Verification items for the finished model (mm, model axes). Face numbers are marked on the shaded views. A direction names the side the tool comes from. Round coordinates to 2 decimals unless told otherwise and drop trailing zeros. Write each loop counter-clockwise with the first axis right and the second up, starting at its lowest first coordinate (ties: lowest second). Pieces come first, ordered by that corner, then holes.
Autodesk Inventor part; units mm, degrees
ref_plane "YZ Plane" through (0, 0, 0) normal (1, 0, 0) x (0, 1, 0)
ref_plane "XZ Plane" through (0, 0, 0) normal (0, 1, 0) x (-1, 0, 0)
ref_plane "XY Plane" through (0, 0, 0) normal (0, 0, 1) x (1, 0, 0)
sketch "Sketch8" plane through (0, 0, 0) normal (0, 0, 1) x (1, 0, 0)
  circle A0 centre (0, 0) radius 15
  dimension "d33" = 30
extrude "Extrusion7" add sketch "Sketch8" against normal blind 8
sketch "Sketch10" plane through (0, 0, -8) normal (0, 0, -1) x (-1, 0, 0)
  line L0 (9, 10.07) -> (-29.1, 10.07)
  arc A0 (10, 9.07) -> (9, 10.07) centre (9, 9.07) ccw
  line L1 (10, 9.07) -> (10, -9.07)
  arc A1 (9, -10.07) -> (10, -9.07) centre (9, -9.07) ccw
  line L2 (-29.1, -10.07) -> (9, -10.07)
  line L3 (-29.1, 10.07) -> (-29.1, -10.07)
  arc A2 (9, -10.47) -> (10.4, -9.07) centre (9, -9.07) ccw
  line L4 (10.4, -9.07) -> (10.4, 9.07)
  arc A3 (10.4, 9.07) -> (9, 10.47) centre (9, 9.07) ccw
  line L5 (9, 10.47) -> (-29.5, 10.47)
  line L6 (-29.5, 10.47) -> (-29.5, -10.47)
  line L7 (-29.5, -10.47) -> (9, -10.47)
  dimension "d59" = 0.4
extrude "Extrusion8" cut sketch "Sketch10" against normal blind 2 contours A0 L1 A1 L2 L3 L0 | L7 L6 L5 A3 L4 A2
sketch "Sketch11" plane through (0, 0, -6) normal (0, 0, -1) x (-1, 0, 0)
  circle A0 centre (0, 0) radius 6.4
  circle A1 centre (0, 0) radius 6.5
  point P0 (0, 0)
  dimension "d58" = 13
extrude "Extrusion9" cut sketch "Sketch11" against normal through all contours A0 | A1
sketch "Sketch13" plane through (0, 0, 0) normal (0, 0, 1) x (1, 0, 0)
  circle A0 centre (0, 0) radius 9.96
  circle A1 centre (0, 0) radius 10.16
  point P0 (0, 0)
  dimension "d44" = 0.2
extrude "Extrusion11" cut sketch "Sketch13" against normal blind 3 contours A0 | A1
sketch "Sketch14" plane through (0, 0, 0) normal (0, 0, 1) x (1, 0, 0)
  circle A0 centre (6.9, 8) radius 0.7835
  circle A1 centre (6.9, -8) radius 0.7835
  circle A2 centre (-8, 8.07) radius 1
  circle A3 centre (-8, -8.07) radius 1
  point P0 (0, 0)
hole "Hole2" at (6.9, 8, 0) at (-8, 8.07, 0) at (-8, -8.07, 0) at (6.9, -8, 0) direction (0, 0, -1) diameter 2.1 end through all
sketch "Sketch15" plane through (0, 0, 0) normal (0, 0, 1) x (1, 0, 0)
  arc A0 (7.3255, 7.0401) -> (5.888, 8.2799) centre (6.9, 8) ccw
  arc A1 (5.888, -8.2799) -> (7.3255, -7.0401) centre (6.9, -8) ccw
  circle A2 centre (-8, 8.07) radius 1.05
  circle A3 centre (-8, -8.07) radius 1.05
  circle A4 centre (6.9, 8) radius 1.9
  circle A5 centre (6.9, -8) radius 1.9
  circle A6 centre (-8, -8.07) radius 1.9
  circle A7 centre (-8, 8.07) radius 1.9
  point P0 (0, 0)
  dimension "d54" = 3.8
extrude "Extrusion12" cut sketch "Sketch15" against normal blind 4.5 contours A2 | A3 | A4 | A5 | A6 | A7
fillet "Fillet2" radius 0.5 8 edges at (5.1562, 8.7544, -1.5) (7.9023, 6.3859, -1.5) (-6.1008, 8.1244, -1.5) (-8.071, 6.1713, -1.5) (-8.071, -6.1713, -1.5) (-6.1008, -8.1244, -1.5) (5.1562, -8.7544, -1.5) (7.9023, -6.3859, -1.5)
properties part number "axis_4_top_frame" material "Aluminum 6061-AHC"
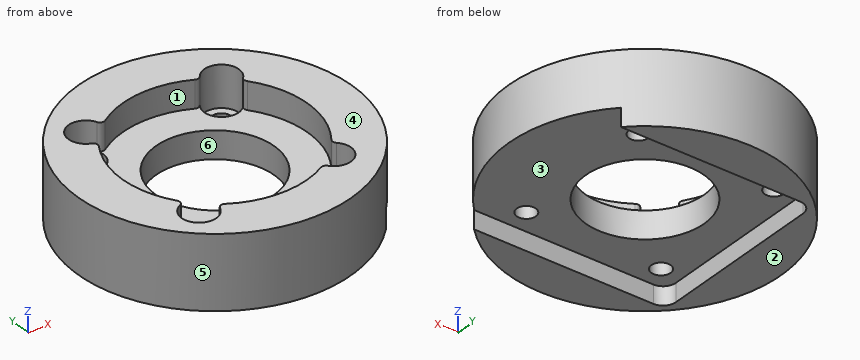
Q1. Sectioned sample at D-D (z = -4). Enter the section's corners in (x, y).
Recorded:
outline: circle Ø30 at (0, 0); hole circle Ø3.8 at (-8, -8.07); hole circle Ø3.8 at (-8, 8.07); hole circle Ø13 at (0, 0); hole circle Ø3.8 at (6.9, -8); hole circle Ø3.8 at (6.9, 8)
Q2. Sectioned sample at A-A (y = 0). Enter the section's corners in (x, z).
Recorded:
outline: (-15, -8) - (-10.4, -8) - (-10.4, -6) - (-6.5, -6) - (-6.5, -3) - (-10.16, -3) - (-10.16, 0) - (-15, 0) - close; (6.5, -6) - (15, -6) - (15, 0) - (10.16, 0) - (10.16, -3) - (6.5, -3) - close
Q3. Sectioned sample at C-C (x = -8). Enter the section's corners in (y, z), plus the area to 3 significant figures.
Recorded:
outline: (-12.69, -8) - (-10.47, -8) - (-10.47, -6) - (-9.12, -6) - (-9.12, -4.5) - (-9.97, -4.5) - (-9.97, 0) - (-12.69, 0) - close; (-7.02, -6) - (7.02, -6) - (7.02, -4.5) - (6.17, -4.5) - (6.17, -3) - (-6.17, -3) - (-6.17, -4.5) - (-7.02, -4.5) - close; (9.12, -6) - (10.47, -6) - (10.47, -8) - (12.69, -8) - (12.69, 0) - (9.97, 0) - (9.97, -4.5) - (9.12, -4.5) - close
area: 83.6 mm2
Q4. Sectioned sample at B-B (x = 0). Enter the section's corners in (y, z), plus the area to 3 significant figures.
Recorded:
outline: (-15, -8) - (-10.47, -8) - (-10.47, -6) - (-6.5, -6) - (-6.5, -3) - (-10.16, -3) - (-10.16, 0) - (-15, 0) - close; (6.5, -6) - (10.47, -6) - (10.47, -8) - (15, -8) - (15, 0) - (10.16, 0) - (10.16, -3) - (6.5, -3) - close
area: 98.2 mm2
Q5. Material ranges on line 1 along X through (y, z) = (-8, -3.75); line 2 along Z through (x, y) = (4.5, 10); line 3 along Z through (x, y) = (-8.5, -2.5), recorded low to high.
Recorded:
line 1: x = -12.69 to -9.9, -6.1 to 5, 8.8 to 12.69
line 2: z = -6 to 0
line 3: z = -6 to -3
Q6. Release check for a two-part mould opening along Y. For the marked faces 4, 5 and 6 record: released by +Y, released by -Y, zero draft, split by the parting line, or undercut.
Recorded:
face 4: zero draft
face 5: split by the parting line
face 6: undercut
Q7. Tool access check on the marked faces 1, 2 and 3. Record the directions out of +Z, -Z, +X, -X, +Y, -Y that give a thin tool (end or side, any length) a straight path to the whole face; none if there is none.
Recorded:
face 1: +Z
face 2: -Z, +X, -X, +Y, -Y
face 3: -Z, +X
Q8. Depth check by flat-ended pin: P1, Ø1, axis at y = -1, z = -7, coming from the +X side; P2, Ø1.3, axis at x = -8, y = 8.07, coming from the -Z side; P3, Ø2.5, axis at x = 6.9, y = -8, coming from the +Z side; P4, Ø1.5, axis at x = 8.5, z = -2, coming from the -Y side. Enter the tip coordinate at first touch or a pass-through.
Recorded:
P1: stops at x = -10.4
P2: passes through
P3: stops at z = -4.5
P4: stops at y = -12.84
